The listing builds one solid part. Answer for the finished solid, in the listing's coordinates (mm). A direction names the side the tool comes from. Coordinates: 2 decimals unless noted, no trailing zeros. Write each loop counter-clockwise with the first axis right and the second up, starting at its lowest first coordinate (ties: lowest second). Pieces come first, ordered by that corner, then holes.
from build123d import *

# Parameters (mm, degrees)
IZIM1_R                     = 36
Y_KSEKLIK_EKSTR_ZYON1_DEPTH = 8
IZIM2_R                     = 3.5
KES_EKSTR_ZYON1_DEPTH       = 8
IZIM3_R                     = 17.5
KES_EKSTR_ZYON2_DEPTH       = 2
IZIM4_W                     = 20
IZIM4_H                     = 29
KES_EKSTR_ZYON3_DEPTH       = 29
KES_EKSTR_ZYON3_DEPTH_BACK  = 6
IZIM5_R                     = 15
Y_KSEKLIK_EKSTR_ZYON2_START = 3
IZIM6_R                     = 20
Y_KSEKLIK_EKSTR_ZYON2_DEPTH = 3
IZIM8_R                     = 12.5
KES_EKSTR_ZYON4_DEPTH       = 3
IZIM13_R                    = 15
KES_EKSTR_ZYON5_DEPTH       = 65
RADYUS2_R                   = 3
RADYUS3_R                   = 3
RADYUS4_R                   = 3


with BuildPart() as part:
    # izim1 → Y_kseklik-Ekstr_zyon1 (new body)
    with BuildSketch(Plane(origin=(0, 0, 0), x_dir=(1, 0, 0), z_dir=(0, 1, 0))):
        with Locations(Location((0, 0, 0), (0, 0, 270))):
            Circle(IZIM1_R)
    extrude(amount=Y_KSEKLIK_EKSTR_ZYON1_DEPTH)

    # izim2 → Kes-Ekstr_zyon1 (cut)
    with BuildSketch(Plane(origin=(0, 8, 0), x_dir=(1, 0, 0), z_dir=(0, 1, 0))):
        with Locations(Location((0, 29, 0), (0, 0, 270))):
            Circle(IZIM2_R)
        with Locations(Location((29, 0, 0), (0, 0, 270))):
            Circle(IZIM2_R)
        with Locations(Location((0, -29, 0), (0, 0, 270))):
            Circle(IZIM2_R)
        with Locations(Location((-29, 0, 0), (0, 0, 270))):
            Circle(IZIM2_R)
    extrude(amount=-KES_EKSTR_ZYON1_DEPTH, mode=Mode.SUBTRACT)

    # izim3 → Kes-Ekstr_zyon2 (cut)
    with BuildSketch(Plane.XZ):
        with Locations(Location((0, 0, 0), (0, 0, 270))):
            Circle(IZIM3_R)
    extrude(amount=-KES_EKSTR_ZYON2_DEPTH, mode=Mode.SUBTRACT)

    # izim4 → D_nd_r1 (revolve)
    with BuildSketch(Plane(origin=(0, 0, 0), x_dir=(0, 0, -1), z_dir=(1, 0, 0)), mode=Mode.PRIVATE) as d_nd_r1_sk:
        with Locations((10, 22.5)):
            Rectangle(IZIM4_W, IZIM4_H)
    revolve(d_nd_r1_sk.sketch.rotate(Axis((0, 37, 0), (0, -1, 0)), 180), axis=Axis((0, 37, 0), (0, -1, 0)))

    # izim5 → Kes-Ekstr_zyon3 (cut, two sides: drawn at the far end of the back side and taken through both)
    with BuildSketch(Plane(origin=(0, 8, 0), x_dir=(1, 0, 0), z_dir=(0, 1, 0)).offset(-KES_EKSTR_ZYON3_DEPTH_BACK)):
        with Locations(Location((0, 0, 0), (0, 0, 270))):
            Circle(IZIM5_R)
    extrude(amount=KES_EKSTR_ZYON3_DEPTH + KES_EKSTR_ZYON3_DEPTH_BACK, mode=Mode.SUBTRACT)

    # izim6 → Y_kseklik-Ekstr_zyon2 (add)
    with BuildSketch(Plane(origin=(0, 37, 0), x_dir=(1, 0, 0), z_dir=(0, 1, 0)).offset(Y_KSEKLIK_EKSTR_ZYON2_START)):
        with Locations(Location((0, 0, 0), (0, 0, 270))):
            Circle(IZIM6_R)
    extrude(amount=-Y_KSEKLIK_EKSTR_ZYON2_DEPTH)

    # izim8 → Kes-Ekstr_zyon4 (cut)
    with BuildSketch(Plane.XZ.offset(-37)):
        with Locations(Location((0, 0, 0), (0, 0, 270))):
            Circle(IZIM8_R)
    extrude(amount=-KES_EKSTR_ZYON4_DEPTH, mode=Mode.SUBTRACT)



with BuildPart() as body_2:
    # izim10 → D_nd_r15 (revolve)
    with BuildSketch(Plane.XY, mode=Mode.PRIVATE) as d_nd_r15_sk:
        with BuildLine():
            Line((0, 95), (0, 97.5))
            ThreePointArc((0, 97.5), (-25.251743677, 80.89033706), (-20, 51.125413912))
            ThreePointArc((-20, 51.125413912), (-10.89033706, 44.748256323), (0, 42.5))
            Line((0, 42.5), (0, 45))
            ThreePointArc((0, 45), (-25, 70), (0, 95))
        make_face()
    revolve(d_nd_r15_sk.sketch.rotate(Axis((0, 97.5, 0), (0, -1, 0)), 180), axis=Axis((0, 97.5, 0), (0, -1, 0)))


with BuildPart() as part_1:
    add(part.part)

    add(body_2.part)  # D_nd_r17 merges body 2
    # izim10_16 → D_nd_r17 (revolve)
    with BuildSketch(Plane.XY, mode=Mode.PRIVATE) as d_nd_r17_sk:
        with BuildLine():
            Line((-20, 51.125413912), (-20, 40))
            Line((-20, 40), (0, 40))
            Line((0, 40), (0, 42.5))
            ThreePointArc((0, 42.5), (-10.89033706, 44.748256323), (-20, 51.125413912))
        make_face()
    revolve(d_nd_r17_sk.sketch.rotate(Axis((0, 97.5, 0), (0, -1, 0)), 270), axis=Axis((0, 97.5, 0), (0, -1, 0)))

    # izim13 → Kes-Ekstr_zyon5 (cut)
    with BuildSketch(Plane.XZ.offset(-40)):
        with Locations(Location((0, 0, 0), (0, 0, 90))):
            Circle(IZIM13_R)
    extrude(amount=-KES_EKSTR_ZYON5_DEPTH, mode=Mode.SUBTRACT)

    # Radyus2
    radyus2_edges = [part_1.edges().sort_by_distance(p)[0] for p in [
        (14.142135624, 51.125413912, 14.142135624),
    ]]
    fillet(radyus2_edges, radius=RADYUS2_R)

    # Radyus3
    # the kernel refuses this fillet: 3 mm, written as the material it adds along each edge
    with BuildSketch(Plane(origin=(0, 40, 0), x_dir=(0, 0, 1), z_dir=(1, 0, 0))) as radyus3_piece_1:
        with BuildLine():
            CenterArc((12, -2.958039892), RADYUS3_R, 0, 80.405931773)
            Line((12.5, 0), (12.51, 0.059160798))
            ThreePointArc((12.51, 0.059160798), (13.75, 0.06), (15, 0.06))
            Line((15, 0.06), (15.06, 0))
            Line((15.06, 0), (15.06, -2.958039892))
            Line((15.06, -2.958039892), (15, -2.958039892))
        make_face()
    revolve(axis=Axis((0, 40, 0), (0, -1, 0)))

    # Radyus4
    radyus4_edges = [part_1.edges().sort_by_distance(p)[0] for p in [
        (0, 8, -20),
    ]]
    fillet(radyus4_edges, radius=RADYUS4_R)


solid = part_1.part
Q1. The part is cut by section A-A, the plane z = 29. Write down the section's boundary in (x, y), then the cut area to 3 significant figures.
Answers below:
outline: (-21.33, 0) - (-3.5, 0) - (-3.5, 8) - (-21.33, 8) - close; (3.5, 0) - (21.33, 0) - (21.33, 8) - (3.5, 8) - close
area: 285 mm2
Q2. The part is cut by section D-D, the plane y = 75. Write down the section's boundary in (x, z).
Answers below:
outline: circle Ø54.08 at (0, 0); hole circle Ø48.99 at (0, 0)
Q3. Determine the mould class of faces 1 (the face through (17, 8, -17)), 2 (the face through (12.3, 37, -3.4)), 3 (the face through (10.81, 3.94, 34.34)) for opening direction Z: released by +Z, released by -Z, zero draft, split by the parting line, or undercut.
Answers below:
face 1: zero draft
face 2: undercut
face 3: split by the parting line
Q4. The part is cut by section C-C, the plane y = 28. Write down the section's boundary in (x, z), then the cut area to 3 significant figures.
Answers below:
outline: circle Ø40 at (0, 0); hole circle Ø30 at (0, 0)
area: 550 mm2
Q5. Which of the six approach directions +Z, -Z, +X, -X, +Y, -Y give full straight-line access (tool end or side, diameter ignored) to faces 4 (the face through (8, 2, -13)), 5 (the face through (-6.007, 30.212, 19.076)), 6 (the face through (14.643, 91.503, -3.252))?
Answers below:
face 4: -Y
face 5: none
face 6: +Y
Q6. Given pin 1 (2 mm diameter, centred on x = 19, y = 37.5, fed in from +Z); pin 2 (6 mm diameter, centred on x = 1.5, z = 22.5, fed in from +Y); pin 3 (12 mm diameter, centred on x = -1.5, y = 29, fed in from +Z), each flat-ended and moving along its own axis, determine where each tip first touches the part or whether it passes through.
Answers below:
pin 1: stops at z = 8.72
pin 2: stops at y = 89.34
pin 3: stops at z = 20
Q7. Find the intervals of material crossed by probe 1 along X at (y, z) = (3, 0); probe 2 along X at (y, z) = (2, -29); probe 3 along Z at (x, y) = (10, 73), in increasing order.
Answers below:
probe 1: x = -36 to -32.5, -25.5 to -15, 15 to 25.5, 32.5 to 36
probe 2: x = -21.33 to -3.5, 3.5 to 21.33
probe 3: z = -25.44 to -22.72, 22.72 to 25.44
Q8. The part is cut by section B-B, the plane x = 29. Write down the section's boundary in (y, z), then the cut area to 3 significant figures.
Answers below:
outline: (0, -21.33) - (8, -21.33) - (8, -3.5) - (0, -3.5) - close; (0, 3.5) - (8, 3.5) - (8, 21.33) - (0, 21.33) - close
area: 285 mm2
